CAD build for the part. Positions are in the model's coordinates, mm. Give positions to 0.01 mm unless a question says otherwise; leave off trailing zeros. Write each loop counter-clockwise with the first axis right and the second up, starting at its lowest first coordinate (ties: lowest second). Pieces come first, ordered by that corner, then holes. Notation, with made-up numbers: (-24, 18) - (24, 18) arc R8 ccw to (24, 26) - close; hole circle Ø7 at (17.5, 18.25). An arc over 180 degrees is marked (long way). Write item = value, one per line. Start each with the question number.
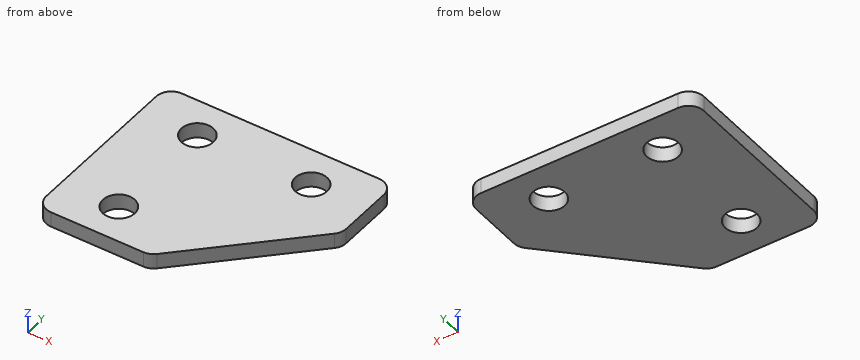
```python
from build123d import *

# Parameters (mm, degrees)
SKETCH_1_W      = 15
SKETCH_1_H      = 25
SKETCH_1_R      = 2.1
SKETCH_1_H_2    = 10
EXTRUDE_1_DEPTH = 2
FILLET_1_R      = 2


with BuildPart() as part:
    # ｽｹｯﾁ1 → ﾎﾞｽ - 押し出し1 (new body)
    # profile 1 of 3: a face of its own
    with BuildSketch(Plane.XY):
        with Locations((0, -7.5)):
            Rectangle(SKETCH_1_W, SKETCH_1_H)
        with Locations((0, -15)):
            Circle(SKETCH_1_R, mode=Mode.SUBTRACT)
        Circle(SKETCH_1_R, mode=Mode.SUBTRACT)
    # profile 2 of 3: a face of its own
    with BuildSketch(Plane.XY):
        Polygon((7.5, -20), (22.5, -5), (7.5, -5), align=None)
    # profile 3 of 3: a face of its own
    with BuildSketch(Plane.XY):
        with Locations((15, 0)):
            Rectangle(SKETCH_1_W, SKETCH_1_H_2)
        with Locations((15, 0)):
            Circle(SKETCH_1_R, mode=Mode.SUBTRACT)
    extrude(amount=EXTRUDE_1_DEPTH)

    # ﾌｨﾚｯﾄ1
    fillet_1_edges = [part.edges().sort_by_distance(p)[0] for p in [
        (7.5, -20, 1),
        (-7.5, -20, 1),
        (-7.5, 5, 1),
        (22.5, 5, 1),
        (22.5, -5, 1),
    ]]
    fillet(fillet_1_edges, radius=FILLET_1_R)


solid = part.part
```
1. Cut at C-C (y = -15). Give the cut face in (x, z).
2. Cut at D-D (y = 0). Give the cut face in (x, z), then the cut area to 3 significant figures.
3. Wall check: line 1 along Y through (x, z) = (0, 0.9); line 2 along X through (y, z) = (1.5, 0.55); line 3 along Y through (x, z) = (20, 0.15). Give the ranges that are in metal, low to high.
4. Cut at A-A (x = 15). Give the cut face in (y, z), then the cut area to 3 significant figures.
5. Cut at B-B (z = 1.15). Give the cut face in (x, y), then the cut area to 3 significant figures.
Output:
q1.outline = (-7.5, 0) - (-2.1, 0) - (-2.1, 2) - (-7.5, 2) - close; (2.1, 0) - (12.5, 0) - (12.5, 2) - (2.1, 2) - close
q2.outline = (-7.5, 0) - (-2.1, 0) - (-2.1, 2) - (-7.5, 2) - close; (2.1, 0) - (12.9, 0) - (12.9, 2) - (2.1, 2) - close; (17.1, 0) - (22.5, 0) - (22.5, 2) - (17.1, 2) - close
q2.area = 43.2 mm2
q3.line_1 = -20 to -17.1, -12.9 to -2.1, 2.1 to 5
q3.line_2 = -7.5 to -1.47, 1.47 to 13.53, 16.47 to 22.5
q3.line_3 = -7.5 to 5
q4.outline = (-12.5, 0) - (-2.1, 0) - (-2.1, 2) - (-12.5, 2) - close; (2.1, 0) - (5, 0) - (5, 2) - (2.1, 2) - close
q4.area = 26.6 mm2
q5.outline = (-7.5, -18) arc R2 ccw to (-5.5, -20) - (6.67, -20) arc R2 ccw to (8.09, -19.41) - (21.91, -5.59) arc R2 ccw to (22.5, -4.17) - (22.5, 3) arc R2 ccw to (20.5, 5) - (-5.5, 5) arc R2 ccw to (-7.5, 3) - close; hole circle Ø4.2 at (0, -15); hole circle Ø4.2 at (0, 0); hole circle Ø4.2 at (15, 0)
q5.area = 593 mm2
